from build123d import *

# Parameters (mm, degrees)
SKETCH_1_W          = 47
SKETCH_1_H          = 20
SKETCH_1_R          = 1.5
SKETCH_1_R_2        = 4.1
EXTRUDE_1_DEPTH     = 6.5
SKETCH_2_W          = 12
SKETCH_2_H          = 3
SKETCH_2_W_2        = 17
SKETCH_2_H_2        = 11
CUT_EXTRUDE_1_DEPTH = 37.976343789
SKETCH_3_R          = 1.25
CUT_EXTRUDE_2_DEPTH = 40.449334595
SKETCH_4_R          = 0.75
CUT_EXTRUDE_3_DEPTH = 37.976343789
CHAMFER_1_SIZE      = 1
SKETCH_5_W          = 2
SKETCH_5_H          = 9
CUT_EXTRUDE_4_DEPTH = 37.976343789


with BuildPart() as part:
    # 草图1 → 凸台-拉伸1 (new body)
    with BuildSketch(Plane(origin=(0, 0, 0), x_dir=(1, 0, 0), z_dir=(0, 1, 0))):
        with Locations((11.5, 0)):
            Rectangle(SKETCH_1_W, SKETCH_1_H)
        with Locations(Location((0, 6, 0), (0, 0, 90))):
            Circle(SKETCH_1_R, mode=Mode.SUBTRACT)
        with Locations(Location((5.196152423, -3, 0), (0, 0, 90))):
            Circle(SKETCH_1_R, mode=Mode.SUBTRACT)
        with Locations(Location((-5.196152423, -3, 0), (0, 0, 90))):
            Circle(SKETCH_1_R, mode=Mode.SUBTRACT)
        with Locations(Location((0, 0, 0), (0, 0, 90))):
            Circle(SKETCH_1_R_2, mode=Mode.SUBTRACT)
    extrude(amount=EXTRUDE_1_DEPTH)

    # 草图2 → 切除-拉伸1 (cut, through all)
    with BuildSketch(Plane(origin=(0, 6.5, 0), x_dir=(1, 0, 0), z_dir=(0, 1, 0))):
        with Locations((27, -8.5)):
            Rectangle(SKETCH_2_W, SKETCH_2_H)
        with Locations((26.5, 4.5)):
            Rectangle(SKETCH_2_W_2, SKETCH_2_H_2)
    extrude(amount=-CUT_EXTRUDE_1_DEPTH, mode=Mode.SUBTRACT)

    # 草图3 → 切除-拉伸2 (cut, through all)
    with BuildSketch(Plane.XY.offset(7)):
        with Locations((23, 3.25)):
            Circle(SKETCH_3_R)
        with Locations((31, 3.25)):
            Circle(SKETCH_3_R)
    extrude(amount=-CUT_EXTRUDE_2_DEPTH, mode=Mode.SUBTRACT)

    # 草图4 → 切除-拉伸3 (cut, through all)
    with BuildSketch(Plane(origin=(0, 6.5, 0), x_dir=(1, 0, 0), z_dir=(0, 1, 0))):
        with Locations(Location((14.5, 3.99875811, 0), (0, 0, 270))):
            Circle(SKETCH_4_R)
    extrude(amount=-CUT_EXTRUDE_3_DEPTH, mode=Mode.SUBTRACT)

    # 倒角1
    chamfer_1_edges = [part.edges().sort_by_distance(p)[0] for p in [
        (18, 3.25, 1),
        (18, 3.25, -10),
    ]]
    chamfer(chamfer_1_edges, length=CHAMFER_1_SIZE)

    # 草图5 → 切除-拉伸4 (cut, through all)
    with BuildSketch(Plane(origin=(0, 6.5, 0), x_dir=(1, 0, 0), z_dir=(0, 1, 0))):
        with Locations((34, -5.5)):
            Rectangle(SKETCH_5_W, SKETCH_5_H)
    extrude(amount=-CUT_EXTRUDE_4_DEPTH, mode=Mode.SUBTRACT)


solid = part.part
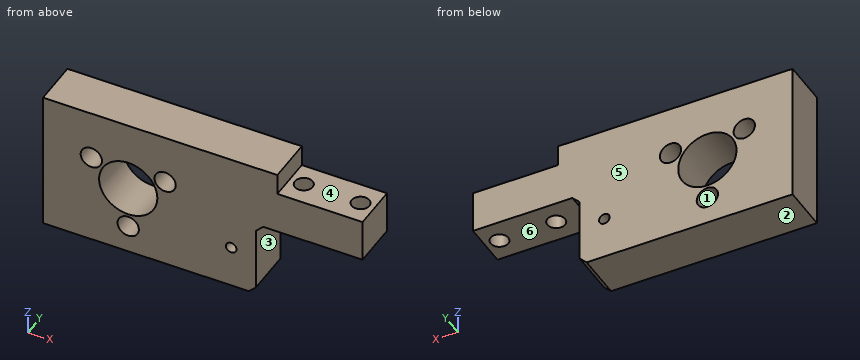
The listing builds one solid part. Answer for the finished solid, in the listing's coordinates (mm). Face numbers are marked on the shaded views. A direction names the side the tool comes from. Round coordinates to 2 decimals unless told otherwise and drop trailing zeros. Write each loop counter-clockwise with the first axis right and the second up, starting at its lowest first coordinate (ties: lowest second). Pieces come first, ordered by that corner, then holes. Notation, with made-up numbers: M -14,23 L 26,23 A20 ccw 26,52 Z; hole C 8,14.5 d8. An arc over 180 degrees is marked long. Write each question's results on one line, items separated by ' | '. Start each with the question number.
(1) The part is cut by section B-B, the plane y = 3.25. Write down the section's boundary in (x, z), and give its area (3 significant figures).
(2) For the marked faces 4, 5 and 6, determine the directions among +Z, -Z, +X, -X, +Y, -Y from which every point of the face is accessible in a straight line to the end or side of a thin tool.
(3) Determine the mould class of the marked faces 1, 2 and 3 for opening direction Z: +Z half, -Z half, draft (parallel to the pull), parting line (faces both ways), or undercut.
(4) Each of these flat-tipped pins is pushed along its axis until it touches: P1, Ø2, axis at x = 23.5, y = 5, coming from the -Z side; P2, Ø0.9, axis at y = 3, z = 8.5, coming from the +X side; P3, Ø2, axis at x = 25, y = 3.5, coming from the +Z side; P4, Ø1.5, axis at x = 31, y = 3.25, coming from the -Z side. Where does it stop, or does it pass through?
(5) The part is cut by section D-D, the plane z = -6. Write down the section's boundary in (x, y), and give its area (4 significant figures).
(6) Find the intervals of material crossed by line 1 (Y direction, x = 23, z = 2.45); line 2 (X direction, y = 4, z = 3); line 3 (Z direction, x = 25.5, y = 1), in increasing order.
(7) The part is cut by section A-A, the plane z = 3. Write down the section's boundary in (x, y), and give its area (3 significant figures).
(8) The part is cut by section C-C, the plane x = 23. Write down the section's boundary in (y, z).
Worked answers:
1) outline: M -12,-10 L 17,-10 L 18,-9 L 18,0 L 19,1 L 21.75,1 L 21.75,7 L 21,7 L 21,10 L -12,10 Z; M 24.25,1 L 29.75,1 L 29.75,7 L 24.25,7 Z; M 32.25,1 L 33,1 L 33,7 L 32.25,7 Z; hole C -5.2,3 d3; hole C 0,0 d8.2; hole C 0,-6 d3; hole C 5.2,3 d3; hole C 14.5,-4 d1.5 | area: 593 mm²
2) face 4: +Z, +X, +Y, -Y | face 5: +Z, -Z, +X, -X, +Y | face 6: -Z, +X, +Y, -Y
3) face 1: undercut | face 2: -Z half | face 3: draft
4) P1: stops at z = 1 | P2: stops at x = 21 | P3: stops at z = 7 | P4: passes through
5) outline: M -12,0 L -1.5,0 L -1.5,6.5 L -12,6.5 Z; M 1.5,0 L 18,0 L 18,6.5 L 1.5,6.5 Z | area: 175.5 mm²
6) line 1: y = 0 to 2, 4.5 to 6.5 | line 2: x = -12 to -6.7, -3.7 to -2.79, 2.79 to 3.7, 6.7 to 22, 24 to 30, 32 to 33 | line 3: z = 1 to 7
7) outline: M -12,0 L -6.7,0 L -6.7,6.5 L -12,6.5 Z; M -3.7,0 L -2.79,0 L -2.79,6.5 L -3.7,6.5 Z; M 2.79,0 L 3.7,0 L 3.7,6.5 L 2.79,6.5 Z; M 6.7,0 L 33,0 L 33,6.5 L 6.7,6.5 Z; hole C 23,3.25 d2.5; hole C 31,3.25 d2.5 | area: 207 mm²
8) outline: M 0,1 L 2,1 L 2,7 L 0,7 Z; M 4.5,1 L 6.5,1 L 6.5,7 L 4.5,7 Z
